Could you check a few things on this model? Use its own coordinates, in mm. Face numbers are marked on the shaded views. A direction names the side the tool comes from. Round coordinates to 2 decimals unless told otherwise and drop trailing zeros. Order: outer loops, then holes, each group sorted by start corner. A loop starts at its lowest first (then second) coordinate and runs counter-clockwise, first axis right, second up.
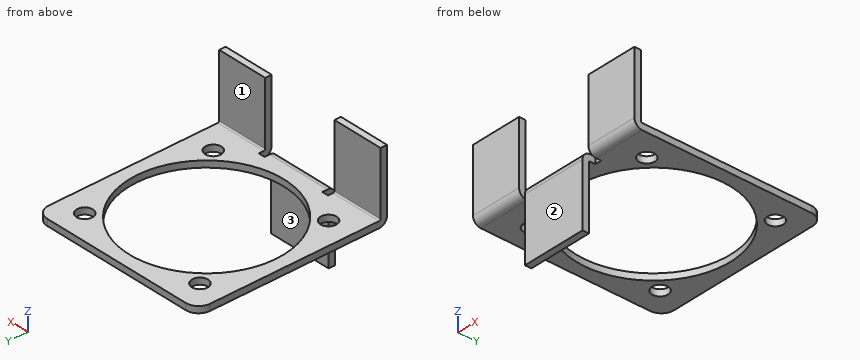
```python
from build123d import *

# Parameters (mm, degrees)
SKIZZE1_W                       = 28
SKIZZE1_H                       = 29.5
SKIZZE1_R                       = 1.25
SKIZZE1_R_2                     = 12
BASIS_BLECH1_DEPTH              = 1
VERRUNDUNG1_R                   = 2
SKIZZE9_W                       = 1
SKIZZE9_H                       = 2
SCHNITT_LINEAR_AUSTRAGEN1_DEPTH = 33.668792448
KANTE_LASCHE2_STRIP_W           = 4.4
KANTE_LASCHE2_STRIP_H           = 1
KANTE_LASCHE2_STRIP_CUT_DEPTH   = 8
KANTE_LASCHE2_STRIP_2_W         = 4.4
KANTE_LASCHE2_STRIP_2_H         = 1
KANTE_LASCHE2_STRIP_CUT_2_DEPTH = 8
KANTE_LASCHE2_DEPTH             = 8
KANTE_LASCHE2_BEND_DEPTH        = 8
KANTE_LASCHE3_STRIP_W           = 4.4
KANTE_LASCHE3_STRIP_H           = 1
KANTE_LASCHE3_STRIP_CUT_DEPTH   = 10
KANTE_LASCHE3_DEPTH             = 10


# Sheet-metal steps are written as plain solids
with BuildPart() as part:
    # Skizze1 → Basis-Blech1 (new body)
    with BuildSketch(Plane.XY):
        with Locations((0, 14.75)):
            Rectangle(SKIZZE1_W, SKIZZE1_H)
        with Locations((-10, 25.5)):
            Circle(SKIZZE1_R, mode=Mode.SUBTRACT)
        with Locations((10, 25.5)):
            Circle(SKIZZE1_R, mode=Mode.SUBTRACT)
        with Locations((10, 5.5)):
            Circle(SKIZZE1_R, mode=Mode.SUBTRACT)
        with Locations((-10, 5.5)):
            Circle(SKIZZE1_R, mode=Mode.SUBTRACT)
        with Locations((0, 15.5)):
            Circle(SKIZZE1_R_2, mode=Mode.SUBTRACT)
    extrude(amount=-BASIS_BLECH1_DEPTH)

    # Verrundung1
    verrundung1_edges = [part.edges().sort_by_distance(p)[0] for p in [
        (-14, 29.5, -0.5),
        (14, 29.5, -0.5),
    ]]
    fillet(verrundung1_edges, radius=VERRUNDUNG1_R)

    # Skizze9 → Schnitt-Linear austragen1 (cut, through all)
    with BuildSketch(Plane.XY):
        with Locations((-5.5, 1)):
            Rectangle(SKIZZE9_W, SKIZZE9_H)
        with Locations((5.5, 1)):
            Rectangle(SKIZZE9_W, SKIZZE9_H)
    extrude(amount=-SCHNITT_LINEAR_AUSTRAGEN1_DEPTH, mode=Mode.SUBTRACT)

    # Kante-Lasche2 strip (across the edge) → Kante-Lasche2 strip cut (cut)
    with BuildSketch(Plane.YZ.offset(-14)):
        with Locations((-1, -0.5)):
            Rectangle(KANTE_LASCHE2_STRIP_W, KANTE_LASCHE2_STRIP_H)
    extrude(amount=KANTE_LASCHE2_STRIP_CUT_DEPTH, mode=Mode.SUBTRACT)

    # Kante-Lasche2 strip 2 (across the edge) → Kante-Lasche2 strip cut 2 (cut)
    with BuildSketch(Plane.YZ.offset(6)):
        with Locations((-1, -0.5)):
            Rectangle(KANTE_LASCHE2_STRIP_2_W, KANTE_LASCHE2_STRIP_2_H)
    extrude(amount=KANTE_LASCHE2_STRIP_CUT_2_DEPTH, mode=Mode.SUBTRACT)

    # Kante-Lasche2 section (across the edge) → Kante-Lasche2 (add)
    with BuildSketch(Plane.YZ.offset(-14)):
        with BuildLine():
            Line((0, 0.2), (0, 10))
            Line((0, 10), (1, 10))
            Line((1, 10), (1, 0.2))
            ThreePointArc((1, 0.2), (1.058578644, 0.058578644), (1.2, 0))
            Line((1.2, 0), (1.2, -1))
            ThreePointArc((1.2, -1), (0.351471863, -0.648528137), (0, 0.2))
        make_face()
    extrude(amount=KANTE_LASCHE2_DEPTH)

    # Kante-Lasche2 section 2 (across the edge) → Kante-Lasche2 bend (add)
    with BuildSketch(Plane.YZ.offset(6)):
        with BuildLine():
            Line((0, 0.2), (0, 10))
            Line((0, 10), (1, 10))
            Line((1, 10), (1, 0.2))
            ThreePointArc((1, 0.2), (1.058578644, 0.058578644), (1.2, 0))
            Line((1.2, 0), (1.2, -1))
            ThreePointArc((1.2, -1), (0.351471863, -0.648528137), (0, 0.2))
        make_face()
    extrude(amount=KANTE_LASCHE2_BEND_DEPTH)

    # Kante-Lasche3 strip (across the edge) → Kante-Lasche3 strip cut (cut)
    with BuildSketch(Plane(origin=(5, 0, -1), x_dir=(0, 1, 0), z_dir=(-1, 0, 0))):
        with Locations((-1, -0.5)):
            Rectangle(KANTE_LASCHE3_STRIP_W, KANTE_LASCHE3_STRIP_H)
    extrude(amount=KANTE_LASCHE3_STRIP_CUT_DEPTH, mode=Mode.SUBTRACT)

    # Kante-Lasche3 section (across the edge) → Kante-Lasche3 (add)
    with BuildSketch(Plane(origin=(5, 0, -1), x_dir=(0, 1, 0), z_dir=(-1, 0, 0))):
        with BuildLine():
            Line((0, 0.2), (0, 10))
            Line((0, 10), (1, 10))
            Line((1, 10), (1, 0.2))
            ThreePointArc((1, 0.2), (1.058578644, 0.058578644), (1.2, 0))
            Line((1.2, 0), (1.2, -1))
            ThreePointArc((1.2, -1), (0.351471863, -0.648528137), (0, 0.2))
        make_face()
    extrude(amount=KANTE_LASCHE3_DEPTH)


solid = part.part
```
Q1. For the marked faces 1, 2 and 3, which set-ups out of +Z, -Z, +X, -X, +Y, -Y let a thin tool reach every point of the face, with its end or its side?
Q2. Imagine slicing it at C-C, the plane x = -10. Please give me the cut outline in (y, z).
Q3. I need wall thicknesses on L1, parallel to Y at x = -10, z = -0.3; L2, parallel to Y at x = -10, z = -0.5; L3, parallel to Y at x = 8.25, z = 6. Which ranges of each line are inside material? Lowest first, please.
Q4. For P1, Ø4, axis at x = -11.5, z = 7.5, coming from the +Y side; P2, Ø0.8, axis at x = -5.5, z = -0.5, coming from the -Y side; P3, Ø8, axis at y = 4.5, z = -8, coming from the +X side, each with a flat end and sliding along its axis, tell me the tip position at first contact or that it passes through.
Q5. Imagine slicing it at D-D, the plane y = 26.25. Please give me the cut outline in (x, z).
Q6. Imagine slicing it at A-A, the plane x = 0. Please give me the cut outline in (y, z), then the cut area to 3 significant figures.
Q7. Imagine slicing it at B-B, the plane y = 15.5. Please give me the cut outline in (x, z), then the cut area to 3 significant figures.
Filled in:
1. face 1: +Z, +X, -X, +Y
1. face 2: +Z, -Z, +X, -X, -Y
1. face 3: -Z, +X, -X, +Y
2. outline: (0, 0.2) arc R1.2 ccw to (1.2, -1) - (4.25, -1) - (4.25, 0) - (1.2, 0) arc R0.2 cw to (1, 0.2) - (1, 10) - (0, 10) - close; (6.75, -1) - (8.87, -1) - (8.87, 0) - (6.75, 0) - close; (22.13, -1) - (24.25, -1) - (24.25, 0) - (22.13, 0) - close; (26.75, -1) - (29.5, -1) - (29.5, 0) - (26.75, 0) - close
3. L1: y = 0.11 to 4.25, 6.75 to 8.87, 22.13 to 24.25, 26.75 to 29.5
3. L2: y = 0.23 to 4.25, 6.75 to 8.87, 22.13 to 24.25, 26.75 to 29.5
3. L3: y = 0 to 1
4. P1: stops at y = 1
4. P2: stops at y = 2
4. P3: stops at x = 5
5. outline: (-14, -1) - (-11, -1) - (-11, 0) - (-14, 0) - close; (-9, -1) - (-5.33, -1) - (-5.33, 0) - (-9, 0) - close; (5.33, -1) - (9, -1) - (9, 0) - (5.33, 0) - close; (11, -1) - (14, -1) - (14, 0) - (11, 0) - close
6. outline: (0, -11) - (1, -11) - (1, -1.2) arc R0.2 cw to (1.2, -1) - (3.5, -1) - (3.5, 0) - (1.2, 0) arc R1.2 ccw to (0, -1.2) - close; (27.5, -1) - (29.5, -1) - (29.5, 0) - (27.5, 0) - close
6. area: 15.2 mm2
7. outline: (-14, -1) - (-12, -1) - (-12, 0) - (-14, 0) - close; (12, -1) - (14, -1) - (14, 0) - (12, 0) - close
7. area: 4.00 mm2
